Geometry: final body of the model. Coordinates: model frame, mm. Coordinates: 2 decimals unless noted, no trailing zeros. Order: outer loops, then holes, each group sorted by start corner. A loop starts at its lowest first (then second) coordinate and runs counter-clockwise, first axis right, second up. Notation, with made-up numbers: (44, 43) -> (48, 43) arc R10 cw to (48, 60) -> close; hole circle Ø1 at (-7, -19.5). An arc over 180 degrees is marked (long way). Answer in a Markdown table with one row per item. Add a question column.
1) Section query A-A on x = 0. Return the cut outline in (y, z) (3 decimals).
2) Ray query, line 1 (X direction, y = 2, z = 97); line 2 (Z direction, x = 1.5, y = 1.75); line 3 (X direction, y = 3, z = -22) (3 decimals). Return the intervals inside material, ascending. Write a range as from..to.
3) Contact query for a flat-ended pin moving along its axis: P1, Ø12, axis at x = -14.5, z = 93, coming from the -Y side. Output: stop coordinate, or through.
4) Section query B-B on z = 106. Return the cut outline in (x, y).
5) Section query C-C on z = -10. Count the separate pieces of the cut face and the enclosed holes in it, then the cut area to 3 significant figures.
6) Section query D-D on x = 10. Return the cut outline in (y, z) (3 decimals).
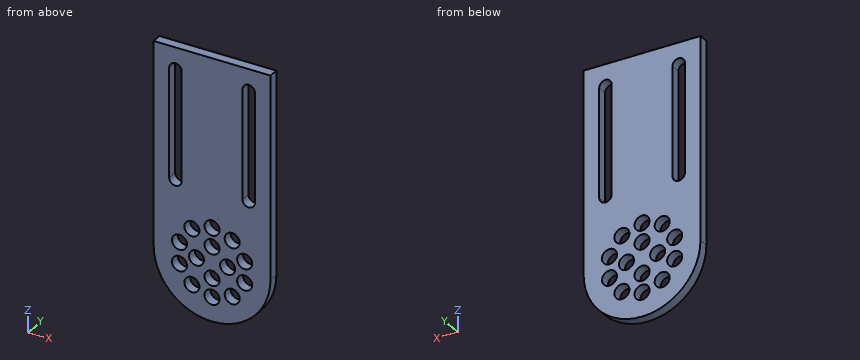
```python
from build123d import *

# Parameters (mm, degrees)
SKETCH1_R           = 4.825
BOSS_EXTRUDE1_DEPTH = 6.35
CUT_EXTRUDE1_DEPTH  = 136.449520117


with BuildPart() as part:
    # Sketch1 → Boss-Extrude1 (new body)
    with BuildSketch(Plane(origin=(0, 0, 0), x_dir=(1, 0, 0), z_dir=(0, 1, 0))):
        with BuildLine():
            Line((-37.5, 0), (-37.5, -130))
            Line((-37.5, -130), (37.5, -130))
            Line((37.5, -130), (37.5, 0))
            ThreePointArc((37.5, 0), (0, 37.5), (-37.5, 0))
        make_face()
        with Locations(Location((0, 22, 0), (0, 0, 270))):
            Circle(SKETCH1_R, mode=Mode.SUBTRACT)
        with Locations(Location((0, 10, 0), (0, 0, 270))):
            Circle(SKETCH1_R, mode=Mode.SUBTRACT)
        with Locations(Location((12.93127555, 17.798373876, 0), (0, 0, 270))):
            Circle(SKETCH1_R, mode=Mode.SUBTRACT)
        with Locations(Location((20.923243358, 6.798373876, 0), (0, 0, 270))):
            Circle(SKETCH1_R, mode=Mode.SUBTRACT)
        with Locations(Location((20.923243358, -6.798373876, 0), (0, 0, 270))):
            Circle(SKETCH1_R, mode=Mode.SUBTRACT)
        with Locations(Location((12.93127555, -17.798373876, 0), (0, 0, 270))):
            Circle(SKETCH1_R, mode=Mode.SUBTRACT)
        with Locations(Location((0, -22, 0), (0, 0, 270))):
            Circle(SKETCH1_R, mode=Mode.SUBTRACT)
        with Locations(Location((-12.93127555, -17.798373876, 0), (0, 0, 270))):
            Circle(SKETCH1_R, mode=Mode.SUBTRACT)
        with Locations(Location((-20.923243358, -6.798373876, 0), (0, 0, 270))):
            Circle(SKETCH1_R, mode=Mode.SUBTRACT)
        with Locations(Location((-20.923243358, 6.798373876, 0), (0, 0, 270))):
            Circle(SKETCH1_R, mode=Mode.SUBTRACT)
        with Locations(Location((-12.93127555, 17.798373876, 0), (0, 0, 270))):
            Circle(SKETCH1_R, mode=Mode.SUBTRACT)
        with Locations(Location((10, 0, 0), (0, 0, 270))):
            Circle(SKETCH1_R, mode=Mode.SUBTRACT)
        with Locations(Location((0, -10, 0), (0, 0, 270))):
            Circle(SKETCH1_R, mode=Mode.SUBTRACT)
        with Locations(Location((-10, 0, 0), (0, 0, 270))):
            Circle(SKETCH1_R, mode=Mode.SUBTRACT)
    extrude(amount=BOSS_EXTRUDE1_DEPTH)

    # Sketch2 → Cut-Extrude1 (cut, through all)
    with BuildSketch(Plane(origin=(0, 6.35, 0), x_dir=(1, 0, 0), z_dir=(0, 1, 0))):
        with BuildLine():
            Line((-27.5, -116), (-27.5, -46))
            ThreePointArc((-27.5, -46), (-23.5, -42), (-19.5, -46))
            Line((-19.5, -46), (-19.5, -116))
            ThreePointArc((-19.5, -116), (-23.5, -120), (-27.5, -116))
        make_face()
    cut_extrude1 = extrude(amount=-CUT_EXTRUDE1_DEPTH, mode=Mode.SUBTRACT)

    # Mirror1: Cut-Extrude1 across plane
    add(cut_extrude1.mirror(Plane(origin=(0, 0, 0), x_dir=(0, 0, 1), z_dir=(1, 0, 0))), mode=Mode.SUBTRACT)


solid = part.part
```
Result:
| question | item | result |
|---|---|---|
| 1 | outline | (0, -37.5) -> (6.35, -37.5) -> (6.35, -26.825) -> (0, -26.825) -> close; (0, -17.175) -> (6.35, -17.175) -> (6.35, -14.825) -> (0, -14.825) -> close; (0, -5.175) -> (6.35, -5.175) -> (6.35, 5.175) -> (0, 5.175) -> close; (0, 14.825) -> (6.35, 14.825) -> (6.35, 17.175) -> (0, 17.175) -> close; (0, 26.825) -> (6.35, 26.825) -> (6.35, 130) -> (0, 130) -> close |
| 2 | line 1 | -37.5..-27.5, -19.5..19.5, 27.5..37.5 |
| 2 | line 2 | -37.47..-26.59, -17.41..-14.59, -5.41..5.41, 14.59..17.41, 26.59..130 |
| 2 | line 3 | -30.369..-15.303, -10.559..-4.825, 4.825..10.559, 15.303..30.369 |
| 3 | P1 | y = 0 |
| 4 | outline | (-37.5, 0) -> (-27.5, 0) -> (-27.5, 6.35) -> (-37.5, 6.35) -> close; (-19.5, 0) -> (19.5, 0) -> (19.5, 6.35) -> (-19.5, 6.35) -> close; (27.5, 0) -> (37.5, 0) -> (37.5, 6.35) -> (27.5, 6.35) -> close |
| 5 | separate pieces | 4 |
| 5 | enclosed holes | 0 |
| 5 | area | 306 mm2 |
| 6 | outline | (0, -36.142) -> (6.35, -36.142) -> (6.35, -21.631) -> (0, -21.631) -> close; (0, -13.966) -> (6.35, -13.966) -> (6.35, -4.825) -> (0, -4.825) -> close; (0, 4.825) -> (6.35, 4.825) -> (6.35, 13.966) -> (0, 13.966) -> close; (0, 21.631) -> (6.35, 21.631) -> (6.35, 130) -> (0, 130) -> close |
